```python
from build123d import *

# Parameters (mm, degrees)
SKETCH_2_W          = 4
SKETCH_2_H          = 52
CUT_EXTRUDE_5_DEPTH = 3.5


with BuildPart() as part:
    # Эскиз1 → Повернуть1 (revolve)
    with BuildSketch(Plane.XY):
        Polygon((24.5, 0), (28.5, 0), (28.5, 2.5), (26, 2.5), (26, 1), (24.5, 1), align=None)
    revolve(axis=Axis((0, 27.258538146, 0), (0, -1, 0)))

    # Эскиз2 → Вырез-Вытянуть5 (cut, through all)
    with BuildSketch(Plane(origin=(0, 0, 0), x_dir=(1, 0, 0), z_dir=(0, 1, 0))):
        with Locations((0, 26)):
            Rectangle(SKETCH_2_W, SKETCH_2_H)
    extrude(amount=CUT_EXTRUDE_5_DEPTH, mode=Mode.SUBTRACT)


solid = part.part
```
Input: part model. Units: mm. Frame: model coordinates. A direction names the side the tool comes from. Round coordinates to 2 decimals unless told otherwise and drop trailing zeros. Loops run counter-clockwise (first coordinate to the right, second up) from the corner with the lowest first, then second, coordinate; pieces in that order, holes last.
1) Pin query (flat end, axial travel): pin 1 (1.2 mm diameter, centred on y = 1, z = -26.5, fed in from +X); pin 2 (1.5 mm diameter, centred on x = -16.5, y = 1, fed in from +Z). Return the tip coordinate at first contact, or that it passes through.
Ans:
pin 1: stops at x = 11.89
pin 2: stops at z = 23.75
2) Set-up query: faces 3 (the flat face through (-13, 0, 21)), 4 (the cylindrical face through (1.115, 1.74, 25.976)), 5 (the flat face through (-2, 1, -27)). Return all of +Z, -Z, +X, -X, +Y, -Y with unobstructed straight access to the full face (end or side cutting, diameter ignored); none if empty.
Ans:
face 3: +Z, -Z, +X, -X, -Y
face 4: +Y
face 5: -Z, +Y, -Y
3) Section query D-D on y = 1.75. Return the cut outline in (x, z), plus the area to 3 significant figures.
Ans:
outline: (-2, -28.43) - (-2, -25.92) arc R26 cw (long way) to (2, -25.92) - (2, -28.43) arc R28.5 ccw (long way) to start
area: 418 mm2
4) Section query A-A on z = -23.5. Return the cut outline in (x, y).
Ans:
outline: (-16.12, 0) - (-6.93, 0) - (-6.93, 1) - (-11.12, 1) - (-11.12, 2.5) - (-16.12, 2.5) - close; (6.93, 0) - (16.12, 0) - (16.12, 2.5) - (11.12, 2.5) - (11.12, 1) - (6.93, 1) - close
5) Pull-direction query (X, two-part tool) for faces 1 (the flat face through (19, 1, 16)), 2 (the flat face through (23.1, 2.5, -12.5)); classes: released by +X, released by -X, zero draft, split by the parting line, or undercut.
Ans:
face 1: undercut
face 2: zero draft
6) Section query B-B on x = 20.5. Return the cut outline in (y, z), plus the area to 3 significant figures.
Ans:
outline: (0, -19.8) - (2.5, -19.8) - (2.5, -15.99) - (1, -15.99) - (1, -13.42) - (0, -13.42) - close; (0, 13.42) - (1, 13.42) - (1, 15.99) - (2.5, 15.99) - (2.5, 19.8) - (0, 19.8) - close
area: 24.2 mm2
7) Section query C-C on x = 0. Return the cut outline in (y, z), plus the area to 3 significant figures.
Ans:
outline: (0, 24.5) - (1, 24.5) - (1, 26) - (2.5, 26) - (2.5, 28.5) - (0, 28.5) - close
area: 7.75 mm2
8) Material intervals for line 1 (X direction, y = 1.85, z = 0); line 2 (X direction, y = 0.3, z = 0); line 3 (Z direction, x = 0, y = 1.6), sorted ascending.
Ans:
line 1: x = -28.5 to -26, 26 to 28.5
line 2: x = -28.5 to -24.5, 24.5 to 28.5
line 3: z = 26 to 28.5
